from build123d import *

# Parameters (mm, degrees)
SKETCH1_W                     = 16
SKETCH1_H                     = 43
BOSS_EXTRUDE1_DEPTH           = 1.6
F_6_0_05_DIAMETER_HOLE1_D     = 1.27
F_6_0_05_DIAMETER_HOLE1_DEPTH = 26.4
F_6_0_05_DIAMETER_HOLE1_TIP   = 0.381546493
SKETCH4_R                     = 1
CUT_EXTRUDE1_DEPTH            = 2.6


with BuildPart() as part:
    # Sketch1 → Boss-Extrude1 (new body)
    with BuildSketch(Plane(origin=(0, 0, 0), x_dir=(1, 0, 0), z_dir=(0, 1, 0))):
        Rectangle(SKETCH1_W, SKETCH1_H)
    extrude(amount=BOSS_EXTRUDE1_DEPTH)

    # #6 (0.05) Diameter Hole1
    with Locations(Plane(origin=(0, 1.6, 0), x_dir=(1, 0, 0), z_dir=(0, 1, 0))):
        with Locations((-6.35, 19.05), (-3.81, 19.05), (-1.27, 19.05), (1.27, 19.05), (3.81, 19.05), (6.35, 19.05), (-3.81, 16.51), (-1.27, 16.51), (1.27, 16.51), (3.81, 16.51), (6.35, 16.51), (-3.81, 13.97), (-1.27, 13.97), (1.27, 13.97), (3.81, 13.97), (6.35, 13.97), (-3.81, 11.43), (-1.27, 11.43), (1.27, 11.43), (3.81, 11.43), (6.35, 11.43), (-3.81, 8.89), (-1.27, 8.89), (1.27, 8.89), (3.81, 8.89), (6.35, 8.89), (-3.81, 6.35), (-1.27, 6.35), (1.27, 6.35), (3.81, 6.35), (6.35, 6.35), (-3.81, 3.81), (-1.27, 3.81), (1.27, 3.81), (3.81, 3.81), (6.35, 3.81), (-3.81, 1.27), (-1.27, 1.27), (1.27, 1.27), (3.81, 1.27), (6.35, 1.27), (-3.81, -1.27), (-1.27, -1.27), (1.27, -1.27), (3.81, -1.27), (6.35, -1.27), (-3.81, -3.81), (-1.27, -3.81), (1.27, -3.81), (3.81, -3.81), (6.35, -3.81), (-3.81, -6.35), (-1.27, -6.35), (1.27, -6.35), (3.81, -6.35), (6.35, -6.35), (-3.81, -8.89), (-1.27, -8.89), (1.27, -8.89), (3.81, -8.89), (6.35, -8.89), (-6.35, 16.51), (-6.35, 13.97), (-6.35, 11.43), (-6.35, 8.89), (-6.35, 6.35), (-6.35, 3.81), (-6.35, 1.27), (-6.35, -1.27), (-6.35, -3.81), (-6.35, -6.35), (-6.35, -8.89), (-6.35, -11.43), (-3.81, -11.43), (-1.27, -11.43), (1.27, -11.43), (3.81, -11.43), (6.35, -11.43), (-6.35, -13.97), (-3.81, -13.97), (-1.27, -13.97), (1.27, -13.97), (3.81, -13.97), (6.35, -13.97), (-6.35, -16.51), (-3.81, -16.51), (-1.27, -16.51), (1.27, -16.51), (3.81, -16.51), (6.35, -16.51), (-6.35, -19.05), (-3.81, -19.05), (-1.27, -19.05), (1.27, -19.05), (3.81, -19.05), (6.35, -19.05)):
            Hole(F_6_0_05_DIAMETER_HOLE1_D / 2, depth=F_6_0_05_DIAMETER_HOLE1_DEPTH)
            with Locations((0, 0, -(F_6_0_05_DIAMETER_HOLE1_DEPTH + F_6_0_05_DIAMETER_HOLE1_TIP / 2))):  # 118° drill point
                Cone(0, F_6_0_05_DIAMETER_HOLE1_D / 2, F_6_0_05_DIAMETER_HOLE1_TIP, mode=Mode.SUBTRACT)

    # Sketch4 → Cut-Extrude1 (cut, through all)
    with BuildSketch(Plane(origin=(0, 1.6, 0), x_dir=(1, 0, 0), z_dir=(0, 1, 0))):
        with Locations((-3.81, 19.05)):
            Circle(SKETCH4_R)
        with Locations((3.81, 19.05)):
            Circle(SKETCH4_R)
        with Locations((-3.81, -19.05)):
            Circle(SKETCH4_R)
        with Locations((3.81, -19.05)):
            Circle(SKETCH4_R)
    extrude(amount=-CUT_EXTRUDE1_DEPTH, mode=Mode.SUBTRACT)


solid = part.part
Geometry check sheet. Reference: the model listing, model coordinates, mm. Coordinates: 2 decimals unless noted, no trailing zeros. Loops run counter-clockwise (first coordinate to the right, second up) from the corner with the lowest first, then second, coordinate; pieces in that order, holes last. Notation, with made-up numbers: (51, 60) - (84, 60) arc R24 cw to (84, 89) - close; hole circle Ø3 at (-5, 50.5). An arc over 180 degrees is marked (long way). Use one line per item in the form item = value. Start each with the question number.
Item 1: Section check A-A, the plane z = 16.51. Enter the section's corners in (x, y) (3 decimals), and give its area (3 significant figures).
Item 2: Thickness scan on probe 1 along Z at (x, y) = (4.5, 0.65). Record the ranges inside material, lowest first.
Item 3: Mould release check, pull along X, two halves, no side actions. Record for faces 1 (the face through (0, 0, 0)), 2 (the face through (-1.19, 0.79, -6.98)), 3 (the face through (-8, 1, 0)), 4 (the face through (-4.151, 0.789, -11.965)): +X half, -X half, draft (parallel to the pull), parting line (faces both ways), or undercut.
Item 4: Section check B-B, the plane x = -3.81. Give the number of separate pieces and of enclosed holes in the cut face, and give its area (3 significant figures).
Computed:
q1.outline = (-8, 0) - (-6.985, 0) - (-6.985, 1.6) - (-8, 1.6) - close; (-5.715, 0) - (-4.445, 0) - (-4.445, 1.6) - (-5.715, 1.6) - close; (-3.175, 0) - (-1.905, 0) - (-1.905, 1.6) - (-3.175, 1.6) - close; (-0.635, 0) - (0.635, 0) - (0.635, 1.6) - (-0.635, 1.6) - close; (1.905, 0) - (3.175, 0) - (3.175, 1.6) - (1.905, 1.6) - close; (4.445, 0) - (5.715, 0) - (5.715, 1.6) - (4.445, 1.6) - close; (6.985, 0) - (8, 0) - (8, 1.6) - (6.985, 1.6) - close
q1.area = 13.4 mm2
q2.probe_1 = -21.5 to -19.77, -18.33 to 18.33, 19.77 to 21.5
q3.face_1 = draft
q3.face_2 = undercut
q3.face_3 = -X half
q3.face_4 = undercut
q4.separate_pieces = 17
q4.enclosed_holes = 0
q4.area = 34.0 mm2
